Autodesk Inventor part; units mm, degrees
ref_plane "YZ Plane" through (0, 0, 0) normal (1, 0, 0) x (0, 1, 0)
ref_plane "XZ Plane" through (0, 0, 0) normal (0, 1, 0) x (-1, 0, 0)
ref_plane "XY Plane" through (0, 0, 0) normal (0, 0, 1) x (1, 0, 0)
ref_plane "РабПлоскость1" through (30.6718, 18.7359, -492.3) normal (0, 0, 1) x (1, 0, 0)
sketch "Эскиз1" plane through (30.6718, 18.7359, -492.3) normal (0, 0, 1) x (1, 0, 0)
  line L0 (9.0963, 0) -> (4.4963, 0)
  line L1 (4.4963, 0) -> (4.4963, -13.5)
  line L2 (9.0963, -13.5) -> (4.4963, -13.5)
  line L3 (9.0963, -13.5) -> (9.0963, 0)
  circle A0 centre (6.7963, -2.75) radius 1.2
  circle A1 centre (6.7963, -10.75) radius 1.2
  line L4 (21.0963, 0) -> (16.4963, 0)
  line L5 (16.4963, 0) -> (16.4963, -13.5)
  line L6 (21.0963, -13.5) -> (16.4963, -13.5)
  line L7 (21.0963, -13.5) -> (21.0963, 0)
  circle A2 centre (18.7963, -2.75) radius 1.2
  circle A3 centre (18.7963, -10.75) radius 1.2
  line L8 (28.0963, 0) -> (23.4963, 0)
  line L9 (23.4963, 0) -> (23.4963, -13.5)
  line L10 (28.0963, -13.5) -> (23.4963, -13.5)
  line L11 (28.0963, -13.5) -> (28.0963, 0)
  circle A4 centre (25.7963, -2.75) radius 1.2
  circle A5 centre (25.7963, -10.75) radius 1.2
  line L12 (40.0963, 0) -> (35.4963, 0)
  line L13 (35.4963, 0) -> (35.4963, -13.5)
  line L14 (40.0963, -13.5) -> (35.4963, -13.5)
  line L15 (40.0963, -13.5) -> (40.0963, 0)
  circle A6 centre (37.7963, -2.75) radius 1.2
  circle A7 centre (37.7963, -10.75) radius 1.2
  circle A8 centre (36.2999, 10.4999) radius 2.5
  circle A9 centre (36.2999, 10.4999) radius 1
  line L16 (-2.7279, 21.2173) -> (47.2721, 21.2173)
  line L17 (47.2721, 21.2173) -> (47.2721, -28.7827)
  line L18 (47.2721, -28.7827) -> (-2.7279, -28.7827)
  line L19 (-2.7279, -28.7827) -> (-2.7279, 21.2173)
  line L20 (22.2721, -16.5) -> (22.2721, -5.5248)
  line L21 (13.8, -23.7827) -> (31.824, -23.7827)
  line L22 (2.2721, 13.0833) -> (42.2721, 13.0833)
  line L23 (2.2721, 7.9833) -> (42.2721, 7.9833)
  circle A10 centre (2.2721, 10.5333) radius 2.55
  circle A11 centre (42.2721, 10.5333) radius 2.55
  point P0 (-30.6718, -18.7359)
  point P1 (-2.7279, -3.7827)
  point P2 (42.2721, 13.0833)
  dimension "d0" = 50
  dimension "d1" = 50
  dimension "d2" = 25
  dimension "d3" = 5
  dimension "d10" = 40
  dimension "d11" = 5
  dimension "d13" = 5
  dimension "d14" = 5.1
extrude "Выдавливание1" add sketch "Эскиз1" along normal blind 4 contours L3 L2 L1 L0 | L7 L6 L5 L4 | L11 L10 L9 L8 | L15 L14 L13 L12 | L16 L17 L18 L19
sketch "Эскиз2" plane through (30.6718, 18.7359, -488.3) normal (0, 0, 1) x (1, 0, 0)
  circle A0 centre (30.2221, -1.7827) radius 1.5
  circle A1 centre (14.3221, -1.7827) radius 1.5
  circle A2 centre (30.2221, -25.7827) radius 1.5
  circle A3 centre (14.3221, -25.7827) radius 1.5
  point P0 (-30.6718, -18.7359)
extrude "Выдавливание2" cut sketch "Эскиз2" against normal blind 10
sketch "Эскиз3" plane through (30.6718, 18.7359, -488.3) normal (0, 0, 1) x (1, 0, 0)
  line L0 (47.2721, 21.2173) -> (-2.7279, 21.2173)
  line L1 (47.2721, -28.7827) -> (47.2721, 21.2173)
  line L2 (-2.7279, 21.2173) -> (47.2721, 21.2173)
  line L3 (47.2721, 21.2173) -> (47.2721, 17.2173)
  line L4 (47.2721, 17.2173) -> (-2.7279, 17.2173)
  line L5 (-2.7279, 17.2173) -> (-2.7279, 21.2173)
  point P0 (-30.6718, -18.7359)
  dimension "d15" = 4
extrude "Выдавливание3" cut sketch "Эскиз3" against normal blind 10
sketch "Эскиз4" plane through (30.6718, 18.7359, -488.3) normal (0, 0, 1) x (1, 0, 0)
  line L0 (-2.7279, 17.2173) -> (-2.7279, -28.7827)
  line L1 (47.2721, 17.2173) -> (-2.7279, 17.2173)
  line L2 (-2.7279, -28.7827) -> (-1.7279, -28.7827)
  line L3 (-1.7279, -28.7827) -> (-1.7279, 17.2173)
  line L4 (-1.7279, 17.2173) -> (-2.7279, 17.2173)
  line L5 (-2.7279, 17.2173) -> (-2.7279, -28.7827)
  line L6 (47.2721, -28.7827) -> (47.2721, 17.2173)
  line L7 (-2.7279, -28.7827) -> (47.2721, -28.7827)
  line L8 (47.2721, 17.2173) -> (46.2721, 17.2173)
  line L9 (46.2721, 17.2173) -> (46.2721, -28.7827)
  line L10 (46.2721, -28.7827) -> (47.2721, -28.7827)
  line L11 (47.2721, -28.7827) -> (47.2721, 17.2173)
  point P0 (-30.6718, -18.7359)
  dimension "d18" = 1
  dimension "d19" = 1
extrude "Выдавливание4" cut sketch "Эскиз4" against normal blind 10 contours L1 L3 L2 L0 | L1 L6 L7 L9
properties part number "деталь на которой рельсы"
CAD build for the part. Positions are in the model's coordinates, mm. A direction names the side the tool comes from. Round coordinates to 2 decimals unless told otherwise and drop trailing zeros. Loops run counter-clockwise (first coordinate to the right, second up) from the corner with the lowest first, then second, coordinate; pieces in that order, holes last.
(1) Cut at B-B (x = 37). Give the cut face in (y, z).
(2) Wall check: line 1 along X through (y, z) = (8, -489.5); line 2 along X through (y, z) = (29.5, -488.7); line 3 along X through (y, z) = (7, -491.45). Give the ranges that are in metal, low to high.
(3) Two-plate mould, pull along X, no slides. Class faces 1 (the flat face through (53, 13, -488.3)), 2 (the flat face through (28.944, 13, -490)), 3 (the cylindrical face through (50.577, 8.446, -490.328)): +X half, -X half, draft (parallel to the pull), parting line (faces both ways), or undercut.
(4) Which spindle directions (+Z, -Z, +X, -X, +Y, -Y) get a long thin tool onto all of the face, cutting with end or side? Do faces 4 (the flat face through (53, 35.953, -490)), 5 (the cylindrical face through (75.493, 29.325, -490.328)). Say none if no direction does.
(5) Cut at A-A (x = 64). Give the cut face in (y, z).
(6) Cut at C-C (z = -491.7). State how many separate pieces and enclosed holes the cut face has, plus the area to 3 significant figures.
Findings below:
1. outline: (-10.05, -492.3) - (6.88, -492.3) - (6.88, -488.3) - (-10.05, -488.3) - close; (9.09, -492.3) - (14.88, -492.3) - (14.88, -488.3) - (9.09, -488.3) - close; (17.09, -492.3) - (26.72, -492.3) - (26.72, -488.3) - (17.09, -488.3) - close; (31.82, -492.3) - (35.95, -492.3) - (35.95, -488.3) - (31.82, -488.3) - close
2. line 1: x = 28.94 to 36.27, 38.67 to 48.27, 50.67 to 55.27, 57.67 to 67.27, 69.67 to 76.94
2. line 2: x = 28.94 to 30.4, 75.48 to 76.94
2. line 3: x = 28.94 to 36.78, 38.15 to 48.78, 50.15 to 55.78, 57.15 to 67.78, 69.15 to 76.94
3. face 1: draft
3. face 2: -X half
3. face 3: undercut
4. face 4: +Z, -Z, +X, -X, +Y
4. face 5: +Z, -Z
5. outline: (-10.05, -492.3) - (26.72, -492.3) - (26.72, -488.3) - (-10.05, -488.3) - close; (31.82, -492.3) - (35.95, -492.3) - (35.95, -488.3) - (31.82, -488.3) - close
6. separate pieces: 1
6. enclosed holes: 13
6. area: 1,920 mm2
